Here's the drawing with two shaded views (mm, measured from the low corner). I have some questions. A direction names the side the tool comes from. Round coordinates to 2 decimals unless told otherwise and drop trailing zeros. Order: outer loops, then holes, each group sorted by start corner. A loop starts at its lowest first (then second) coordinate and runs counter-clockwise, first axis right, second up. Notation, with made-up numbers: (50, -38) - (97, -38) arc R34 cw to (97, 1) - close; hole circle Ø2 at (78, 24.25). An arc over 180 degrees is marked (long way). One line per item, written item: value.
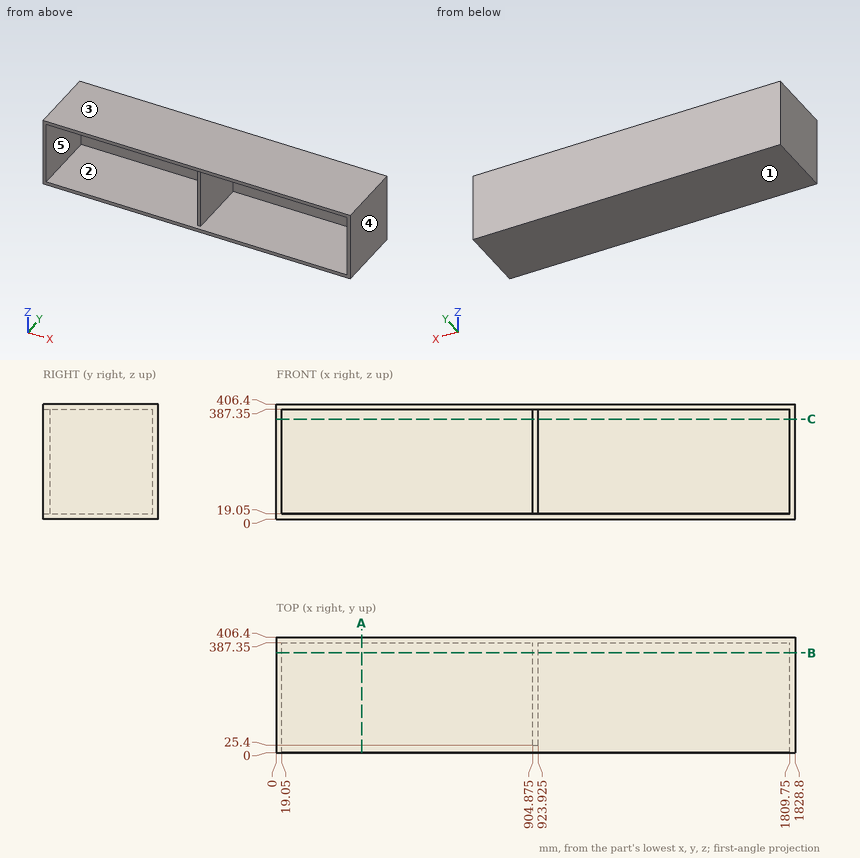
Q1. If I drill on line 1 along X through (y, z) = (305, 69) (3 decimals); line 2 along Z through (x, y) = (731, 225), over which ranges is the centre line in solid material (lowest first)?
Results list:
line 1: 0 to 19.05, 904.875 to 923.925, 1809.75 to 1828.8
line 2: 0 to 19.05, 387.35 to 406.4
Q2. We'd pull the mould along Z, two halves only. Please class the marked faces 1, 2 and 3: released by +Z, released by -Z, zero draft, split by the parting line, or undercut.
Results list:
face 1: released by -Z
face 2: undercut
face 3: released by +Z
Q3. If we section it at B-B, the plane y = 351: Please give me the cut outline in (x, z) (3 decimals).
Results list:
outline: (0, 0) - (1828.8, 0) - (1828.8, 406.4) - (0, 406.4) - close; hole (19.05, 19.05) - (904.875, 19.05) - (904.875, 387.35) - (19.05, 387.35) - close; hole (923.925, 19.05) - (1809.75, 19.05) - (1809.75, 387.35) - (923.925, 387.35) - close
Q4. Which directions (+Z, -Z, +X, -X, +Y, -Y) give clear straight access to the entire face, cutting with the end or side of a thin tool? Please do the marked faces 4 and 5.
Results list:
face 4: +Z, -Z, +X, +Y, -Y
face 5: -Y
Q5. If we section it at C-C, the plane z = 353.5: Please give me the cut outline in (x, y) (3 decimals).
Results list:
outline: (0, 0) - (19.05, 0) - (19.05, 387.35) - (904.875, 387.35) - (904.875, 25.4) - (923.925, 25.4) - (923.925, 387.35) - (1809.75, 387.35) - (1809.75, 0) - (1828.8, 0) - (1828.8, 406.4) - (0, 406.4) - close
Q6. Will these pins go through, and if not, where does the flat tip stop? pin 1 (4 mm diameter, centred on x = 1059, z = 336.5, fed in from -Y); pin 2 (9.5 mm diameter, centred on x = 913, z = 219, fed in from -Y); pin 3 (3 mm diameter, centred on x = 1071, z = 247.5, fed in from -Y).
Results list:
pin 1: y = 387.35
pin 2: y = 25.4
pin 3: y = 387.35
Q7. If we section it at A-A, the plane x = 300.5: Please give me the cut outline in (y, z), then the cut area to 3 significant figures.
Results list:
outline: (0, 0) - (406.4, 0) - (406.4, 406.4) - (0, 406.4) - (0, 387.35) - (387.35, 387.35) - (387.35, 19.05) - (0, 19.05) - close
area: 22,500 mm²
